Source: CAD feature listing. Evaluate the final solid. Frame: model axes, mm. Face numbers are marked on the shaded views. Round coordinates to 2 decimals unless told otherwise and drop trailing zeros. Loops run counter-clockwise (first coordinate to the right, second up) from the corner with the lowest first, then second, coordinate; pieces in that order, holes last. Notation, with made-up numbers: (10, 87) -> (51, 87) arc R13 ccw to (51, 97) -> close; hole circle Ø11 at (-0.75, 5.5). An arc over 180 degrees is marked (long way). Write item = value, one per line.
from build123d import *

# Parameters (mm, degrees)
SKETCH1_R           = 152.4
BOSS_EXTRUDE1_DEPTH = 63.5
SKETCH2_R           = 150.8125
CUT_EXTRUDE1_DEPTH  = 49.2125
SKETCH3_W           = 1.5875
SKETCH3_H           = 101.6
CUT_REVOLVE1_ANGLE  = 75
SKETCH4_R           = 19.05
CUT_EXTRUDE2_DEPTH  = 2.54


with BuildPart() as part:
    # Sketch1 → Boss-Extrude1 (new body, symmetric)
    with BuildSketch(Plane(origin=(0, 0, 0), x_dir=(1, 0, 0), z_dir=(0, 1, 0))):
        Circle(SKETCH1_R)
    extrude(amount=BOSS_EXTRUDE1_DEPTH, both=True)

    # Sketch2 → Cut-Extrude1 (cut, symmetric)
    with BuildSketch(Plane(origin=(0, 0, 0), x_dir=(1, 0, 0), z_dir=(0, 1, 0))):
        Circle(SKETCH2_R)
    extrude(amount=CUT_EXTRUDE1_DEPTH, both=True, mode=Mode.SUBTRACT)

    # Sketch3 → Cut-Revolve1 (revolve, symmetric, cut)
    with BuildSketch(Plane(origin=(0, 0, 0), x_dir=(0, 0, -1), z_dir=(1, 0, 0))) as cut_revolve1_sk:
        with Locations((-151.60625, 0)):
            Rectangle(SKETCH3_W, SKETCH3_H)
    revolve(axis=Axis((0, 0, 0), (0, 1, 0)), revolution_arc=CUT_REVOLVE1_ANGLE / 2, mode=Mode.SUBTRACT)
    revolve(cut_revolve1_sk.sketch, axis=Axis((0, 0, 0), (0, -1, 0)), revolution_arc=CUT_REVOLVE1_ANGLE / 2, mode=Mode.SUBTRACT)

    # Sketch4 → Cut-Extrude2 (cut)
    with BuildSketch(Plane(origin=(0, 63.5, 0), x_dir=(1, 0, 0), z_dir=(0, 1, 0))):
        Circle(SKETCH4_R)
    extrude(amount=-CUT_EXTRUDE2_DEPTH, mode=Mode.SUBTRACT)


solid = part.part
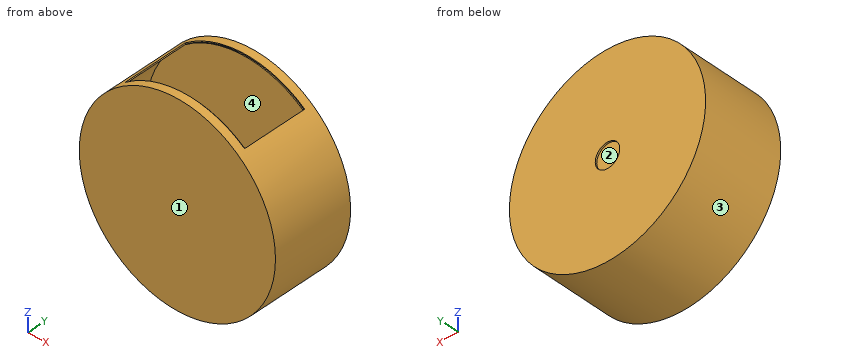
1. Section query B-B (x = 0). Return the cut outline in (y, z).
Evaluation:
outline = (-63.5, -152.4) -> (63.5, -152.4) -> (63.5, -19.05) -> (60.96, -19.05) -> (60.96, 19.05) -> (63.5, 19.05) -> (63.5, 152.4) -> (50.8, 152.4) -> (50.8, 150.81) -> (49.21, 150.81) -> (49.21, -150.81) -> (-49.21, -150.81) -> (-49.21, 150.81) -> (-50.8, 150.81) -> (-50.8, 152.4) -> (-63.5, 152.4) -> close
2. Mould query, pull axis Z, two halves, no side actions, for the marked faces 1, 2, 3 and 4. Classes: released by +Z, released by -Z, zero draft, split by the parting line, or undercut.
Evaluation:
face_1 = zero draft
face_2 = undercut
face_3 = split by the parting line
face_4 = undercut
3. Contact query for flat-ended pins moving along their axis: pin 1 Ø12 at (y, z) = (-30, -96) entering from -X; pin 2 Ø10 at (x, y) = (39.5, -6.5) entering from +Z; pin 3 Ø1 at (y, z) = (20, -64.5) entering from +X. Output: stop coordinate, or through.
Evaluation:
pin_1 = -122.99
pin_2 = -144.1
pin_3 = 138.31
4. Line query: probe 1 along Y at (x, z) = (-34.5, 1.5); probe 2 along X at (y, z) = (62.3, 0); probe 3 along Y at (x, z) = (13, -9.5). Output: solid intervals per line, ascending. Write a range as from..to.
Evaluation:
probe_1 = -63.5..-49.21, 49.21..63.5
probe_2 = -152.4..-19.05, 19.05..152.4
probe_3 = -63.5..-49.21, 49.21..60.96
5. Section query D-D (z = 35). Return the cut outline in (x, y).
Evaluation:
outline = (-148.33, -63.5) -> (148.33, -63.5) -> (148.33, 63.5) -> (-148.33, 63.5) -> close; hole (-146.69, -49.21) -> (146.69, -49.21) -> (146.69, 49.21) -> (-146.69, 49.21) -> close
6. Section query C-C (x = 105). Return the cut outline in (y, z), then the cut area to 3 significant figures.
Evaluation:
outline = (-63.5, -110.46) -> (63.5, -110.46) -> (63.5, 110.46) -> (-63.5, 110.46) -> close; hole (-49.21, -108.26) -> (49.21, -108.26) -> (49.21, 108.26) -> (-49.21, 108.26) -> close
area = 6,750 mm²
7. Section query A-A (z = 0). Return the cut outline in (x, y).
Evaluation:
outline = (-152.4, -63.5) -> (152.4, -63.5) -> (152.4, 63.5) -> (19.05, 63.5) -> (19.05, 60.96) -> (-19.05, 60.96) -> (-19.05, 63.5) -> (-152.4, 63.5) -> close; hole (-150.81, -49.21) -> (150.81, -49.21) -> (150.81, 49.21) -> (-150.81, 49.21) -> close
